```python
from build123d import *

# Parameters (mm, degrees)
F0_W     = 500
F0_H     = 800
F0_R     = 7.5
F0_R_2   = 4.5
F1_DEPTH = 10
F3_DEPTH = 500
F5_DEPTH = 500.001


with BuildPart() as f1:
    # F0 (on Top) → F1 (new body)
    with BuildSketch(Plane.XY):
        with Locations((0, -175)):
            Rectangle(F0_W, F0_H)
        with Locations((-175, -461)):
            Circle(F0_R, mode=Mode.SUBTRACT)
        with Locations((175, -461)):
            Circle(F0_R, mode=Mode.SUBTRACT)
        with Locations((-217.5, 15)):
            Circle(F0_R_2, mode=Mode.SUBTRACT)
        with Locations((-132.5, 15)):
            Circle(F0_R_2, mode=Mode.SUBTRACT)
        with BuildLine():
            ThreePointArc((-200, 170), (-198.5355339059, 173.5355339059), (-195, 175))
            Line((-195, 175), (-155, 175))
            ThreePointArc((-155, 175), (-151.4644660941, 173.5355339059), (-150, 170))
            Line((-150, 170), (-150, -30))
            ThreePointArc((-150, -30), (-151.4644660941, -33.5355339059), (-155, -35))
            Line((-155, -35), (-195, -35))
            ThreePointArc((-195, -35), (-198.5355339059, -33.5355339059), (-200, -30))
            Line((-200, -30), (-200, 170))
        make_face(mode=Mode.SUBTRACT)
        with Locations((-217.5, 125)):
            Circle(F0_R_2, mode=Mode.SUBTRACT)
        with Locations((-132.5, 125)):
            Circle(F0_R_2, mode=Mode.SUBTRACT)
        with Locations((132.5, 15)):
            Circle(F0_R_2, mode=Mode.SUBTRACT)
        with Locations((217.5, 15)):
            Circle(F0_R_2, mode=Mode.SUBTRACT)
        with BuildLine():
            Line((195, -35), (155, -35))
            ThreePointArc((155, -35), (151.4644660941, -33.5355339059), (150, -30))
            Line((150, -30), (150, 170))
            ThreePointArc((150, 170), (151.4644660941, 173.5355339059), (155, 175))
            Line((155, 175), (195, 175))
            ThreePointArc((195, 175), (198.5355339059, 173.5355339059), (200, 170))
            Line((200, 170), (200, -30))
            ThreePointArc((200, -30), (198.5355339059, -33.5355339059), (195, -35))
        make_face(mode=Mode.SUBTRACT)
        with Locations((132.5, 125)):
            Circle(F0_R_2, mode=Mode.SUBTRACT)
        with Locations((217.5, 125)):
            Circle(F0_R_2, mode=Mode.SUBTRACT)
    extrude(amount=F1_DEPTH)

    # F2 (on face) → F3 (join, through all)
    with BuildSketch(Plane.YZ.offset(250)):
        with BuildLine():
            Line((-150, 30), (-200, 30))
            ThreePointArc((-200, 30), (-203.5355339059, 28.5355339059), (-205, 25))
            Line((-205, 25), (-205, 15))
            ThreePointArc((-205, 15), (-206.4644660941, 11.4644660941), (-210, 10))
            Line((-210, 10), (-195, 10))
            Line((-195, 10), (-195, 15))
            ThreePointArc((-195, 15), (-193.5355339059, 18.5355339059), (-190, 20))
            Line((-190, 20), (-160, 20))
            ThreePointArc((-160, 20), (-156.4644660941, 18.5355339059), (-155, 15))
            Line((-155, 15), (-155, 10))
            Line((-155, 10), (-140, 10))
            ThreePointArc((-140, 10), (-143.5355339059, 11.4644660941), (-145, 15))
            Line((-145, 15), (-145, 25))
            ThreePointArc((-145, 25), (-146.4644660941, 28.5355339059), (-150, 30))
        make_face()
    extrude(amount=-F3_DEPTH)

    # F4 (on face) → F5 (cut, through all)
    with BuildSketch(Plane.YZ.offset(250)):
        Polygon((-150, 0), (-200, 0), (-211.0108286142, 0), (-211.0108286142, -10.5340015143), (-138.8553231955, -10.5340015143), (-138.8553231955, 0), align=None)
        with BuildLine():
            Line((-155, 10), (-195, 10))
            Line((-195, 10), (-195, 5))
            ThreePointArc((-195, 5), (-196.4644660941, 1.4644660941), (-200, 0))
            Line((-200, 0), (-150, 0))
            ThreePointArc((-150, 0), (-153.5355339059, 1.4644660941), (-155, 5))
            Line((-155, 5), (-155, 10))
        make_face()
    extrude(amount=-F5_DEPTH, mode=Mode.SUBTRACT)


solid = f1.part
```
Part model, mm, in its own coordinate system. A direction names the side the tool comes from. Round coordinates to 2 decimals unless told otherwise and drop trailing zeros. Write each loop counter-clockwise with the first axis right and the second up, starting at its lowest first coordinate (ties: lowest second). Pieces come first, ordered by that corner, then holes. Notation, with made-up numbers: M -28.75,-36 L -14.75,-36 A11 cw -14.75,-31 Z; hole C 19,11.5 d10. An arc over 180 degrees is marked long. Answer as CSV lines item,"result". Start each with the question number.
1) Band-saw the part on A-A (y = 41). List the corners of the cut face in (x, z), then the cut area to 3 significant figures.
2) Band-saw the part on C-C (y = -232). List the corners of the cut face in (x, z), then the cut area to 3 significant figures.
3) Drop flat-ended pins along their axis: pin 1 (9 mm diameter, centred on x = 75.5, y = -181.5, fed in from -Z); pin 2 (14.5 mm diameter, centred on x = -132.5, y = 15, fed in from +Z); pin 3 (5 mm diameter, centred on x = -10, z = 25.5, fed in from +Y). Give the stop position or say it passes through.
4) Drill centre lines: L1, parallel to Y at x = -132.5, z = 4; L2, parallel to Y at x = -217.5, z = 6.5; L3, parallel to Y at x = -29, z = 4.25. Where is each one in solid material? Low to high.
5) Band-saw the part on B-B (x = -10.5). List the corners of the cut face in (y, z).
6) Mould opens along Y. For faces 1 (the face through (-3, 45, 10)), 2 (the face through (181.93, -463.87, 4.93)), 3 (the face through (4, -175, 20)) say: +Y half, -Y half, draft (parallel to the pull), parting line (faces both ways), or undercut.
7) Which spindle directions (+Z, -Z, +X, -X, +Y, -Y) get a long thin tool onto all of the face, cutting with end or side? Do faces 4 (the face through (-250, -177, 22)), 5 (the face through (-3, -390, 10)). Say none if no direction does.
Worked out:
1,outline,"M -250,0 L -200,0 L -200,10 L -250,10 Z; M -150,0 L 150,0 L 150,10 L -150,10 Z; M 200,0 L 250,0 L 250,10 L 200,10 Z"
1,area,"4,000 mm²"
2,outline,"M -250,0 L 250,0 L 250,10 L -250,10 Z"
2,area,"5,000 mm²"
3,pin 1,"z = 20"
3,pin 2,"z = 10"
3,pin 3,"y = -145"
4,L1,"-575 to -195.1, -154.9 to 10.5, 19.5 to 120.5, 129.5 to 225"
4,L2,"-575 to -195, -155 to 10.5, 19.5 to 120.5, 129.5 to 225"
4,L3,"-575 to -195.06, -154.94 to 225"
5,outline,"M -575,0 L -200,0 A5 ccw -195,5 L -195,15 A5 cw -190,20 L -160,20 A5 cw -155,15 L -155,5 A5 ccw -150,0 L 225,0 L 225,10 L -140,10 A5 cw -145,15 L -145,25 A5 ccw -150,30 L -200,30 A5 ccw -205,25 L -205,15 A5 cw -210,10 L -575,10 Z"
6,face 1,"draft"
6,face 2,"undercut"
6,face 3,"undercut"
7,face 4,"+Z, -Z, -X, +Y, -Y"
7,face 5,"+Z, +X, -X, -Y"
